```python
from build123d import *

# Parameters (mm, degrees)
SKETCH009_W  = 20
SKETCH009_H  = 54
SKETCH009_R  = 1.1
PAD009_DEPTH = 0.3
FILLET_R     = 5
SKETCH001_W  = 1.6
SKETCH001_H  = 0.7
PAD001_DEPTH = 1.3
FILLET001_R  = 0.15
FILLET002_R  = 0.15


with BuildPart() as fillet_body:
    # Sketch009 → Pad009 (new body)
    with BuildSketch(Plane.XY):
        with Locations((10, 27)):
            Rectangle(SKETCH009_W, SKETCH009_H)
        with Locations((10, 52)):
            Circle(SKETCH009_R, mode=Mode.SUBTRACT)
        with Locations((10, 2)):
            Circle(SKETCH009_R, mode=Mode.SUBTRACT)
        Polygon((1, 48), (1, 6), (2.325, 6), (2.325, 20.15), (3.925, 20.15), (3.925, 6), (5.075, 6), (5.075, 22.75), (6.675, 22.75), (6.675, 6), (7.825, 6), (7.825, 20.15), (9.425, 20.15), (9.425, 6), (10.575, 6), (10.575, 22.75), (12.175, 22.75), (12.175, 6), (13.325, 6), (13.325, 20.15), (14.925, 20.15), (14.925, 6), (16.075, 6), (16.075, 22.75), (17.675, 22.75), (17.675, 6), (19, 6), (19, 48), (17.675, 48), (17.675, 33.85), (16.075, 33.85), (16.075, 48), (14.925, 48), (14.925, 31.25), (13.325, 31.25), (13.325, 48), (12.175, 48), (12.175, 33.85), (10.575, 33.85), (10.575, 48), (9.425, 48), (9.425, 31.25), (7.825, 31.25), (7.825, 48), (6.675, 48), (6.675, 33.85), (5.075, 33.85), (5.075, 48), (3.925, 48), (3.925, 31.25), (2.325, 31.25), (2.325, 48), align=None, mode=Mode.SUBTRACT)
    extrude(amount=PAD009_DEPTH)

    # Fillet
    fillet_edges = [fillet_body.edges().sort_by_distance(p)[0] for p in [
        (20, 0, 0.15),
        (0, 0, 0.15),
        (20, 54, 0.15),
        (0, 54, 0.15),
    ]]
    fillet(fillet_edges, radius=FILLET_R)


with BuildPart() as fusion:
    # Sketch001 → Pad001 (new body)
    with BuildSketch(Plane.XY.offset(0.3)):
        with Locations((3.125, 19.8)):
            Rectangle(SKETCH001_W, SKETCH001_H)
        with Locations((5.875, 22.4)):
            Rectangle(SKETCH001_W, SKETCH001_H)
        with Locations((8.625, 19.8)):
            Rectangle(SKETCH001_W, SKETCH001_H)
        with Locations((11.375, 22.4)):
            Rectangle(SKETCH001_W, SKETCH001_H)
        with Locations((14.125, 19.8)):
            Rectangle(SKETCH001_W, SKETCH001_H)
        with Locations((16.875, 22.4)):
            Rectangle(SKETCH001_W, SKETCH001_H)
        with Locations((3.125, 31.6)):
            Rectangle(SKETCH001_W, SKETCH001_H)
        with Locations((5.875, 34.2)):
            Rectangle(SKETCH001_W, SKETCH001_H)
        with Locations((8.625, 31.6)):
            Rectangle(SKETCH001_W, SKETCH001_H)
        with Locations((11.375, 34.2)):
            Rectangle(SKETCH001_W, SKETCH001_H)
        with Locations((14.125, 31.6)):
            Rectangle(SKETCH001_W, SKETCH001_H)
        with Locations((16.875, 34.2)):
            Rectangle(SKETCH001_W, SKETCH001_H)
    extrude(amount=PAD001_DEPTH)

    # Fillet001
    fillet001_edges = [fusion.edges().sort_by_distance(p)[0] for p in [
        (9.425, 19.45, 0.95),
        (8.625, 19.45, 1.6),
        (7.825, 19.45, 0.95),
        (7.825, 31.25, 0.95),
        (8.625, 31.25, 1.6),
        (9.425, 31.25, 0.95),
        (10.575, 22.75, 0.95),
        (11.375, 22.75, 1.6),
        (12.175, 22.75, 0.95),
        (16.075, 22.05, 0.95),
        (16.875, 22.05, 1.6),
        (17.675, 22.05, 0.95),
        (13.325, 31.95, 0.95),
        (14.125, 31.95, 1.6),
        (14.925, 31.95, 0.95),
        (5.075, 33.85, 0.95),
        (5.875, 33.85, 1.6),
        (6.675, 33.85, 0.95),
    ]]
    fillet(fillet001_edges, radius=FILLET001_R)

    # Fillet002
    fillet002_edges = [fusion.edges().sort_by_distance(p)[0] for p in [
        (3.925, 19.45, 0.95),
        (3.125, 19.45, 1.6),
        (2.325, 19.45, 0.95),
        (13.325, 19.45, 0.95),
        (14.125, 19.45, 1.6),
        (14.925, 19.45, 0.95),
        (2.325, 31.95, 0.95),
        (3.125, 31.95, 1.6),
        (3.925, 31.95, 0.95),
        (5.075, 22.75, 0.95),
        (5.875, 22.75, 1.6),
        (6.675, 22.75, 0.95),
        (16.075, 33.85, 0.95),
        (16.875, 33.85, 1.6),
        (17.675, 33.85, 0.95),
        (12.175, 33.85, 0.95),
        (11.375, 33.85, 1.6),
        (10.575, 33.85, 0.95),
    ]]
    fillet(fillet002_edges, radius=FILLET002_R)

    # Fusion: union Fillet body
    add(fillet_body.part)


solid = fusion.part
```
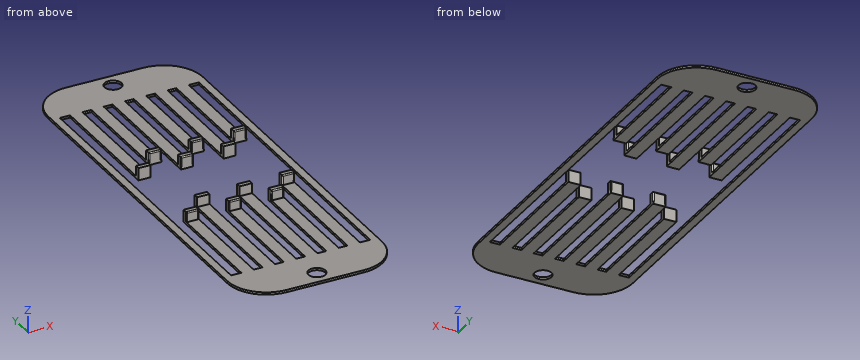
Design review of the part built by this model. Coordinates are the model's own, in mm. Round coordinates to 2 decimals unless told otherwise and drop trailing zeros. Write each loop counter-clockwise with the first axis right and the second up, starting at its lowest first coordinate (ties: lowest second). Pieces come first, ordered by that corner, then holes. Notation, with made-up numbers: (10, 13.5) -> (65, 13.5) arc R22 cw to (65, 40.5) -> close; hole circle Ø3 at (-29, 58.5). An arc over 180 degrees is marked (long way). Write item = value, one per line. Start each with the question number.
1) Take a section at A-A, the plane x = 10. State the section outline as (y, z) points, plus the area to 3 significant figures.
2) Take a section at B-B, the plane y = 2. State the section outline as (x, z) points, plus the area to 3 significant figures.
3) Take a section at C-C, the plane x = 6. State the section outline as (y, z) points.
4) Clearance check with flat-ended pins moving along their axes: pin 1 (0.8 mm diameter, centred on y = 37, z = 1, fed in from +X); pin 2 (0.9 mm diameter, centred on x = 8.5, z = 1, fed in from -Y); pin 3 (3 mm diameter, centred on x = 5.5, y = 5.5, fed in from -Z); pin 4 (1 mm diameter, centred on x = 13.5, y = 43.5, fed in from +Z). State where each tip first meets the part, or that it passes through.
5) Take a section at D-D, the plane y = 47. Count the separate pieces of the cut face and the enclosed holes in it, plus the area to 3 significant figures.
6) Wall thickness on probe 1 along Y at (x, z) = (10, 0.15); probe 2 along X at (y, z) = (34, 1.4) (3 decimals); probe 3 along X at (y, z) = (33, 0.25) (3 decimals): over which ranges is each line inside the solid? List them lowest first. Write a range as from..to.
Results list:
q1.outline = (0, 0) -> (0.9, 0) -> (0.9, 0.3) -> (0, 0.3) -> close; (3.1, 0) -> (6, 0) -> (6, 0.3) -> (3.1, 0.3) -> close; (48, 0) -> (50.9, 0) -> (50.9, 0.3) -> (48, 0.3) -> close; (53.1, 0) -> (54, 0) -> (54, 0.3) -> (53.1, 0.3) -> close
q1.area = 2.28 mm²
q2.outline = (1, 0) -> (8.9, 0) -> (8.9, 0.3) -> (1, 0.3) -> close; (11.1, 0) -> (19, 0) -> (19, 0.3) -> (11.1, 0.3) -> close
q2.area = 4.74 mm²
q3.outline = (0, 0) -> (22.75, 0) -> (22.75, 1.45) arc R0.15 ccw to (22.6, 1.6) -> (22.05, 1.6) -> (22.05, 0.3) -> (0, 0.3) -> close; (33.85, 0) -> (54, 0) -> (54, 0.3) -> (34.55, 0.3) -> (34.55, 1.6) -> (34, 1.6) arc R0.15 ccw to (33.85, 1.45) -> close
q4.pin_1 = through
q4.pin_2 = 19.45
q4.pin_3 = 0
q4.pin_4 = 0.3
q5.separate_pieces = 8
q5.enclosed_holes = 0
q5.area = 3.48 mm²
q6.probe_1 = 0..0.9, 3.1..6, 48..50.9, 53.1..54
q6.probe_2 = 5.075..6.675, 10.575..12.175, 16.075..17.675
q6.probe_3 = 0..1, 2.325..3.925, 7.825..9.425, 13.325..14.925, 19..20
